Part model, mm, in its own coordinate system. Give positions to 0.01 mm unless a question says otherwise; leave off trailing zeros. Order: outer loops, then holes, each group sorted by start corner. A loop starts at its lowest first (then second) coordinate and runs counter-clockwise, first axis right, second up.
from build123d import *

# Parameters (mm, degrees)
ESQUISSE1_W             = 300
ESQUISSE1_H             = 70
BOSS_EXTRU_1_DEPTH      = 5
CONG_2_R                = 2
CONG_3_R                = 2
ESQUISSE2_W             = 10
ESQUISSE2_H             = 60
ENL_V_MAT_EXTRU_1_DEPTH = 155.110350074


with BuildPart() as part:
    # Esquisse1 → Boss.-Extru.1 (new body)
    with BuildSketch(Plane.XY):
        Rectangle(ESQUISSE1_W, ESQUISSE1_H)
    extrude(amount=BOSS_EXTRU_1_DEPTH)

    # Congé2
    cong_2_edges = [part.edges().sort_by_distance(p)[0] for p in [
        (0, 35, 0),
    ]]
    fillet(cong_2_edges, radius=CONG_2_R)

    # Congé3
    cong_3_edges = [part.edges().sort_by_distance(p)[0] for p in [
        (0, 35, 5),
    ]]
    fillet(cong_3_edges, radius=CONG_3_R)

    # Esquisse2 → Enlèv. mat.-Extru.1 (cut, through all)
    with BuildSketch(Plane(origin=(0, 0, 0), x_dir=(-1, 0, 0), z_dir=(0, 0, -1))):
        with Locations((-35, -5)):
            Rectangle(ESQUISSE2_W, ESQUISSE2_H)
        with Locations((35, -5)):
            Rectangle(ESQUISSE2_W, ESQUISSE2_H)
    extrude(amount=-ENL_V_MAT_EXTRU_1_DEPTH, mode=Mode.SUBTRACT)


solid = part.part
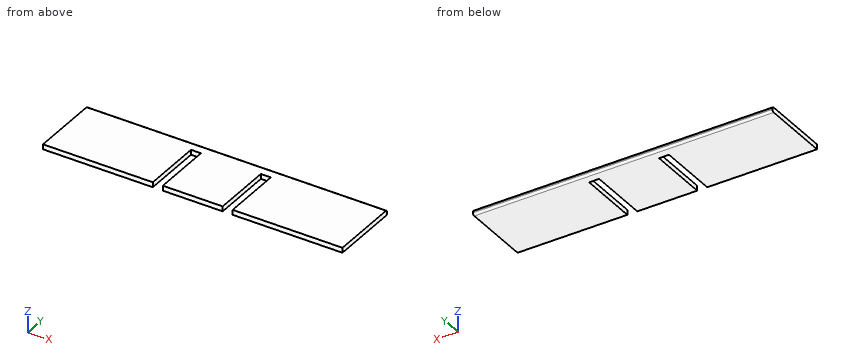
Item 1: Drill centre lines: probe 1 along X at (y, z) = (-6.5, 3.5); probe 2 along Y at (x, z) = (29, 1.75); probe 3 along Y at (x, z) = (46, 1.45). Where is each one in solid material? Low to high.
Item 2: Band-saw the part on B-B on z = 1. List the corners of the cut face in (x, y), plus the area to 3 significant figures.
Item 3: Band-saw the part on A-A on y = -27.5. List the corners of the cut face in (x, z).
Working result:
1. probe 1: x = -150 to -40, -30 to 30, 40 to 150
1. probe 2: y = -35 to 34.98
1. probe 3: y = -35 to 34.92
2. outline: (-150, -35) - (-40, -35) - (-40, 25) - (-30, 25) - (-30, -35) - (30, -35) - (30, 25) - (40, 25) - (40, -35) - (150, -35) - (150, 34.73) - (-150, 34.73) - close
2. area: 19,700 mm2
3. outline: (-150, 0) - (-40, 0) - (-40, 5) - (-150, 5) - close; (-30, 0) - (30, 0) - (30, 5) - (-30, 5) - close; (40, 0) - (150, 0) - (150, 5) - (40, 5) - close
